Autodesk Inventor part; units mm, degrees
ref_plane "Plano inicial" through (0, 0, -50) normal (0, 0, 1) x (1, 0, 0)
ref_plane "Plano final" through (0, 0, 175) normal (0, 0, 1) x (1, 0, 0)
ref_plane "Plano de trabalho5" through (-15, -10, 175) normal (0, 0, 1) x (1, 0, 0)
ref_plane "Plano inicial" through (0, 0, -50) normal (0, 0, 1) x (1, 0, 0)
ref_plane "Plano final" through (0, 0, 175) normal (0, 0, 1) x (1, 0, 0)
sketch "Esboço" plane through (0, 0, 0) normal (0, 0, 1) x (1, 0, 0)
  line L0 (-15, -21.25) -> (-15, 21.25)
  line L1 (-11.25, 25) -> (11.25, 25)
  line L2 (15, 21.25) -> (15, -21.25)
  line L3 (11.25, -25) -> (-11.25, -25)
  arc A0 (-15, -21.25) -> (-11.25, -25) centre (-11.25, -21.25) ccw
  arc A1 (-11.25, 25) -> (-15, 21.25) centre (-11.25, 21.25) ccw
  arc A2 (15, 21.25) -> (11.25, 25) centre (11.25, 21.25) ccw
  arc A3 (11.25, -25) -> (15, -21.25) centre (11.25, -21.25) ccw
  arc A4 (-11.25, 22.5) -> (-12.5, 21.25) centre (-11.25, 21.25) ccw
  line L4 (-11.25, 22.5) -> (11.25, 22.5)
  arc A5 (12.5, 21.25) -> (11.25, 22.5) centre (11.25, 21.25) ccw
  line L5 (12.5, 21.25) -> (12.5, -21.25)
  arc A6 (11.25, -22.5) -> (12.5, -21.25) centre (11.25, -21.25) ccw
  line L6 (11.25, -22.5) -> (-11.25, -22.5)
  arc A7 (-12.5, -21.25) -> (-11.25, -22.5) centre (-11.25, -21.25) ccw
  line L7 (-12.5, -21.25) -> (-12.5, 21.25)
  line L8 (0, 36.0873) -> (0, -36.0873) construction
  line L9 (-22.0873, 0) -> (22.0873, 0) construction
  dimension "d7" = 3.75
  dimension "d10" = 50
  dimension "d11" = 30
  dimension "d12" = 2.5
  dimension "d15" = 25
  dimension "d16" = 15
extrude "Corpo" add sketch "Esboço" along normal up to surface (225 mm away) from surface at -50
sketch "Sketch3" plane through (0, 0, 0) normal (0, 0, 1) x (1, 0, 0)
  line L0 (0, 0) -> (10, 0)
ref_plane "Work Plane3" through (0, 0, 0) normal (0, -1, 0) x (1, 0, 0)
sketch "Sketch4" plane through (0, 0, 0) normal (0, -1, 0) x (1, 0, 0)
  line L0 (-2, -50) -> (12, -50)
  line L1 (-2, 175) -> (12, 175)
  dimension "d18" = 225
ref_plane "Plano de trabalho5" through (-15, -10, 175) normal (0, 0, 1) x (1, 0, 0)
split "Dividir2" plane through (-15, -10, 175) removes the side toward (0, 0, 1)
ref_plane "Plano de trabalho6" through (-2.5, -25, -50) normal (0, 0.7071, -0.7071) x (1, 0, 0)
split "Dividir3" plane through (-2.5, -25, -50) removes the side toward (0, 0.7071, -0.7071)
ref_plane "Plano de trabalho7" through (0, -25, 175) normal (0, 0.7071, 0.7071) x (1, 0, 0)
split "Dividir4" plane through (0, -25, 175) removes the side toward (0, 0.7071, 0.7071)
equation "\"d7\" = G_IR"
equation "\"d10\" = G_H"
equation "\"d11\" = G_W"
equation "\"d12\" = G_T"
equation "\"d15\" = 0.5 * d10"
equation "\"d16\" = 0.5 * d11"
equation "\"d3\" = G_L"
equation "\"G_W\" = 30"
equation "\"G_H\" = 50"
equation "\"G_T\" = 2.5"
equation "\"G_IR\" = 3.75"
equation "\"G_L\" = d18"
equation "\"G_OFFSET_END\" = 0"
equation "\"d14\" = G_OFFSET_END + B_L"
equation "\"B_L\" = 175"
properties part number "ISO 12633-2 - 50x30x2.5 - 225" material "Aço, suave"
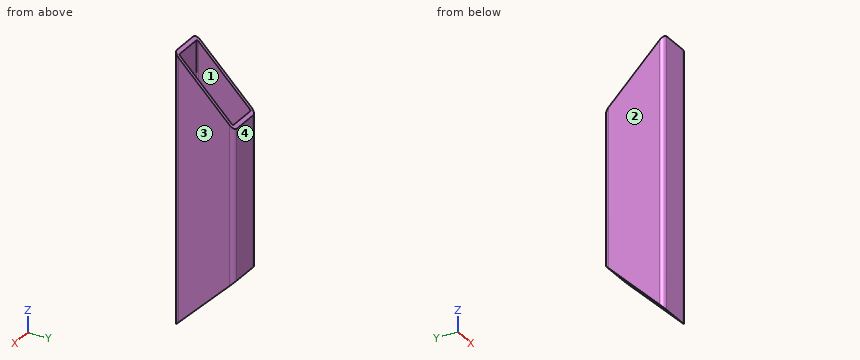
Can you work these out from the model? Positions are in its coordinate system, mm. Face numbers are marked on the shaded views. Coordinates: 2 decimals unless noted, no trailing zeros. Order: outer loops, then holes, each group sorted by start corner. A loop starts at its lowest first (then second) coordinate and runs counter-clockwise, first axis right, second up.
1. If we section it at A-A (y = 1.5): Please give me the cut outline in (x, z).
2. I need wall thicknesses on line 1 (Y direction, x = 10.75, z = 91); line 2 (X direction, y = -14.5, z = 77); line 3 (Y direction, x = 8, z = -7). Which ranges of each line are inside material? Lowest first, please.
3. If we section it at B-B (x = 7): Please give me the cut outline in (y, z), then the cut area to 3 significant figures.
4. If we section it at D-D (z = 150.5): Please give me the cut outline in (x, y), then the cut area to 3 significant figures.
5. I'm going to push a flat-ended pin straight in: pin 1 (6 mm diameter, centred on y = 13, z = -17.5, fed in from -X). Where does the tip first touch, or does it pass through?
6. If we section it at C-C (z = 70.5): Please give me the cut outline in (x, y), then the cut area to 3 significant figures.
7. Thinking about a two-plate mould opening in X: for the marked faces 1, 2, 3 and 4, which applies, +X half, -X half, draft (parallel to the pull), parting line (faces both ways), or undercut?
Entries:
1. outline: (-15, -23.5) - (-12.5, -23.5) - (-12.5, 148.5) - (-15, 148.5) - close; (12.5, -23.5) - (15, -23.5) - (15, 148.5) - (12.5, 148.5) - close
2. line 1: y = -25 to -22.5, 22.5 to 25
2. line 2: x = -15 to -12.5, 12.5 to 15
2. line 3: y = -25 to -22.5
3. outline: (-25, -50) - (-22.5, -47.5) - (-22.5, 172.5) - (-25, 175) - close; (22.5, -2.5) - (25, 0) - (25, 125) - (22.5, 127.5) - close
3. area: 875 mm2
4. outline: (-15, -21.25) arc R3.75 ccw to (-11.25, -25) - (11.25, -25) arc R3.75 ccw to (15, -21.25) - (15, -0.5) - (12.5, -0.5) - (12.5, -21.25) arc R1.25 cw to (11.25, -22.5) - (-11.25, -22.5) arc R1.25 cw to (-12.5, -21.25) - (-12.5, -0.5) - (-15, -0.5) - close
4. area: 180 mm2
5. pin 1: passes through
6. outline: (-15, -21.25) arc R3.75 ccw to (-11.25, -25) - (11.25, -25) arc R3.75 ccw to (15, -21.25) - (15, 21.25) arc R3.75 ccw to (11.25, 25) - (-11.25, 25) arc R3.75 ccw to (-15, 21.25) - close; hole (-12.5, -21.25) arc R1.25 ccw to (-11.25, -22.5) - (11.25, -22.5) arc R1.25 ccw to (12.5, -21.25) - (12.5, 21.25) arc R1.25 ccw to (11.25, 22.5) - (-11.25, 22.5) arc R1.25 ccw to (-12.5, 21.25) - close
6. area: 364 mm2
7. face 1: undercut
7. face 2: -X half
7. face 3: +X half
7. face 4: draft
